```python
from build123d import *

# Parameters (mm, degrees)
F0_W     = 64
F0_H     = 47
F1_DEPTH = 2
F2_D     = 3.5
F3_R     = 17.5
F4_DEPTH = 25


with BuildPart() as f1:
    # F0 (on Front) → F1 (new body)
    with BuildSketch(Plane.XZ):
        Rectangle(F0_W, F0_H)
    extrude(amount=F1_DEPTH)

    # F2 (through all)
    with Locations(Plane(origin=(0, 0, 0), x_dir=(1, 0, 0), z_dir=(0, 1, 0))):
        with Locations((-29.35, 17.15), (-19.9, 19.75), (19.9, 19.75), (29.35, 17.15), (29.35, -17.15), (19.9, -19.75), (-19.9, -19.75), (-29.35, -17.15)):
            Hole(F2_D / 2)

    # F3 (on face) → F4 (cut)
    with BuildSketch(Plane.XZ.offset(2)):
        Circle(F3_R)
    extrude(amount=-F4_DEPTH, mode=Mode.SUBTRACT)


solid = f1.part
```
Part model, mm, in its own coordinate system. Round coordinates to 2 decimals unless told otherwise and drop trailing zeros. Write each loop counter-clockwise with the first axis right and the second up, starting at its lowest first coordinate (ties: lowest second). Pieces come first, ordered by that corner, then holes.
Item 1: Two-plate mould, pull along Z, no slides. Class faces 1 (the flat face through (0, -1, -23.5)), 2 (the flat face through (-8, -2, 16)), 3 (the cylindrical face through (-30.967, -1.014, 17.82)): +Z half, -Z half, draft (parallel to the pull), parting line (faces both ways), or undercut.
Results:
face 1: -Z half
face 2: draft
face 3: undercut
Item 2: Cut at B-B, the plane x = 29.35. Give the cut face in (y, z), plus the area to 3 significant figures.
Results:
outline: (-2, -23.5) - (0, -23.5) - (0, -18.9) - (-2, -18.9) - close; (-2, -15.4) - (0, -15.4) - (0, 15.4) - (-2, 15.4) - close; (-2, 18.9) - (0, 18.9) - (0, 23.5) - (-2, 23.5) - close
area: 80.0 mm2
Item 3: Cut at C-C, the plane y = -0.9. Count the separate pieces of the cut face and the enclosed holes in it, plus the area to 3 significant figures.
Results:
separate pieces: 1
enclosed holes: 9
area: 1,970 mm2
Item 4: Cut at D-D, the plane x = -1.5. Give the cut face in (y, z).
Results:
outline: (-2, -23.5) - (0, -23.5) - (0, -17.44) - (-2, -17.44) - close; (-2, 17.44) - (0, 17.44) - (0, 23.5) - (-2, 23.5) - close
Item 5: Probe L1, parallel to X at y = -1.2, z = 19.75; L2, parallel to Z at x = -19.9, y = -0.6; L3, parallel to Z at x = 0, y = -0.95. List the from-to ranges inside material, lowest first.
Results:
L1: x = -32 to -21.65, -18.15 to 18.15, 21.65 to 32
L2: z = -23.5 to -21.5, -18 to 18, 21.5 to 23.5
L3: z = -23.5 to -17.5, 17.5 to 23.5
Item 6: Cut at A-A, the plane z = 19.75. Give the cut face in (x, y), plus the area to 3 significant figures.
Results:
outline: (-32, -2) - (-21.65, -2) - (-21.65, 0) - (-32, 0) - close; (-18.15, -2) - (18.15, -2) - (18.15, 0) - (-18.15, 0) - close; (21.65, -2) - (32, -2) - (32, 0) - (21.65, 0) - close
area: 114 mm2
